Here's how the part is built. I have some questions about the finished solid (model axes, mm). A direction names the side the tool comes from. Give positions to 0.01 mm unless a question says otherwise; leave off trailing zeros. Loops run counter-clockwise (first coordinate to the right, second up) from the corner with the lowest first, then second, coordinate; pieces in that order, holes last. Notation, with made-up numbers: (26.5, 28.25) - (69.5, 28.25) arc R25 cw to (69.5, 66.25) - close; hole circle Ø8 at (75.25, 67.5). An arc over 180 degrees is marked (long way). Use a Markdown table: item, result.
from build123d import *

# Parameters (mm, degrees)
F1_DEPTH = 25


with BuildPart() as f1:
    # F0 (on Top) → F1 (new body)
    with BuildSketch(Plane.XY):
        with BuildLine():
            ThreePointArc((52.7247383893, 0), (45.7247383893, 7), (38.7247383893, 0))
            Line((38.7247383893, 0), (40.7247383893, 0))
            ThreePointArc((40.7247383893, 0), (45.7247383893, 5), (50.7247383893, 0))
            ThreePointArc((50.7247383893, 0), (49.2602722952, -3.5355339059), (45.7247383893, -5))
            Line((45.7247383893, -5), (45.7247383893, -7))
            ThreePointArc((45.7247383893, -7), (50.6744858576, -4.9497474683), (52.7247383893, 0))
        make_face()
        with BuildLine():
            ThreePointArc((0, -5), (3.5355339059, -3.5355339059), (5, 0))
            ThreePointArc((5, 0), (-3.5355339059, 3.5355339059), (0, -5))
        make_face()
        with BuildLine():
            Line((22.8623691946, 0), (5, 0))
            ThreePointArc((5, 0), (3.5355339059, -3.5355339059), (0, -5))
            Line((0, -5), (45.1135477291, -6.9732665213))
            ThreePointArc((45.1135477291, -6.9732665213), (40.5634238948, -4.7287242137), (38.7247383893, 0))
            Line((38.7247383893, 0), (22.8623691946, 0))
        make_face()
        with BuildLine():
            Line((45.7247383893, -7), (45.1135477291, -6.9732665213))
            ThreePointArc((45.1135477291, -6.9732665213), (45.4188508683, -6.9933134367), (45.7247383893, -7))
        make_face()
        with BuildLine():
            ThreePointArc((38.7247383893, 0), (40.5634238948, -4.7287242137), (45.1135477291, -6.9732665213))
            Line((45.1135477291, -6.9732665213), (45.7247383893, -7))
            Line((45.7247383893, -7), (45.7247383893, -5))
            ThreePointArc((45.7247383893, -5), (42.1892044833, -3.5355339059), (40.7247383893, 0))
            Line((40.7247383893, 0), (38.7247383893, 0))
        make_face()
    extrude(amount=F1_DEPTH)


solid = f1.part
(1) If I drill on line 1 (X direction, y = 3, z = 4.25); line 2 (X direction, y = 1, z = 6); line 3 (X direction, y = -3, z = 17.5), over which ranges is the centre line in solid material (lowest first)?
A:
| item | result |
|---|---|
| line 1 | -4 to 4, 39.4 to 41.72, 49.72 to 52.05 |
| line 2 | -4.9 to 4.9, 38.8 to 40.83, 50.62 to 52.65 |
| line 3 | -4 to 41.72, 49.72 to 52.05 |
(2) We'd pull the mould along X, two halves only. Please class faces 3 (the face through (22.241, -5.973, 12.325)), 4 (the face through (23, -3, 25)), 5 (the face through (-3, 4, 12)): pulls with the +X half, pulls with the -X half, needs draft (parallel to the pull), parting line crosses it, or undercut.
A:
| item | result |
|---|---|
| face 3 | pulls with the -X half |
| face 4 | needs draft |
| face 5 | undercut |
(3) On a 3-axis mill with a long thin cutter (end or side, diameter ignored), from which of +Z, -Z, +X, -X, +Y, -Y can I reach the whole of each face in a straight line? I mean faces 1 (the face through (23, -3, 0)), 2 (the face through (22, 0, 12)). Say none if no direction works.
A:
| item | result |
|---|---|
| face 1 | -Z, +X, -X, +Y, -Y |
| face 2 | +Z, -Z, +Y |
(4) Suppose I cut it at B-B on x = 44. Write out the boundary of the cut face in (y, z), plus the area to 3 significant figures.
A:
| item | result |
|---|---|
| outline | (-6.92, 0) - (-4.69, 0) - (-4.69, 25) - (-6.92, 25) - close; (4.69, 0) - (6.78, 0) - (6.78, 25) - (4.69, 25) - close |
| area | 108 mm2 |
(5) Suppose I cut it at D-D on y = 4.25. Write out the boundary of the cut face in (x, z), plus the area to 3 significant figures.
A:
| item | result |
|---|---|
| outline | (-2.63, 0) - (2.63, 0) - (2.63, 25) - (-2.63, 25) - close; (40.16, 0) - (43.09, 0) - (43.09, 25) - (40.16, 25) - close; (48.36, 0) - (51.29, 0) - (51.29, 25) - (48.36, 25) - close |
| area | 278 mm2 |
(6) Will these pins go through, and if not, where does the flat tip stop? pin 1 (1.5 mm diameter, centred on x = 6.5, z = 3, fed in from -Y); pin 2 (8 mm diameter, centred on x = 1, z = 15, fed in from -Y); pin 3 (12.5 mm diameter, centred on x = 17, z = 17, fed in from +Y).
A:
| item | result |
|---|---|
| pin 1 | y = -5.32 |
| pin 2 | y = -5.22 |
| pin 3 | y = 0 |
(7) Suppose I cut it at A-A on z = 22.75. Write out the boundary of the cut face in (x, y), plus the area to 3 significant figures.
A:
| item | result |
|---|---|
| outline | (0, -5) - (45.11, -6.97) arc R7 ccw (long way) to (38.72, 0) - (5, 0) arc R5 ccw (long way) to start; hole circle Ø10 at (45.72, 0) |
| area | 370 mm2 |
(8) Suppose I cut it at C-C on y = -1.75. Write out the boundary of the cut face in (x, z).
A:
| item | result |
|---|---|
| outline | (-4.68, 0) - (41.04, 0) - (41.04, 25) - (-4.68, 25) - close; (50.41, 0) - (52.5, 0) - (52.5, 25) - (50.41, 25) - close |
